Could you check a few things on this model? Use its own coordinates, in mm. A direction names the side the tool comes from. Coordinates: 2 decimals unless noted, no trailing zeros. Order: outer loops, then holes, each group sorted by start corner. A loop starts at its lowest first (then second) coordinate and runs counter-clockwise, first axis right, second up. Notation, with made-up numbers: (37.25, 1.25) -> (60.25, 1.25) arc R22 ccw to (60.25, 36.25) -> close; hole circle Ø4 at (23, -9). An arc over 180 degrees is marked (long way). Put each result on its own line as item: value. Start each with the question number.
Q1. Will these pins go through, and if not, where does the flat tip stop? pin 1 (6 mm diameter, centred on x = 15.5, y = -10.5, fed in from -Z); pin 2 (2 mm diameter, centred on y = -1, z = 1, fed in from -X); pin 3 (1.5 mm diameter, centred on x = 28, z = 0.5, fed in from -Y).
Q2. If we section it at A-A (y = 0): Please give me the cut outline in (x, z).
Q3. For faces 1 (the face through (-15, 7, 0)), 2 (the face through (0, 5, -5)), 3 (the face through (-15, -7, 0)), which set-ups out of +Z, -Z, +X, -X, +Y, -Y let a thin tool reach every point of the face, with its end or its side?
Q4. If we section it at B-B (x = -7.5): Please give me the cut outline in (y, z).
Q5. If we section it at D-D (x = 6.5): Please give me the cut outline in (y, z).
Q6. We'd pull the mould along X, two halves only. Please class faces 4 (the face through (-18, 7, 0)), 5 (the face through (39, 0, 0)), 6 (the face through (-7.605, -6.244, -0.275)): +X half, -X half, draft (parallel to the pull), parting line (faces both ways), or undercut.
Q7. If we section it at C-C (z = 0): Please give me the cut outline in (x, y).
Q8. Please list where these lines run through material, in increasing order: line 1 along X through (y, z) = (5, 5); line 2 along Y through (x, z) = (1.5, 1.5); line 3 along Y through (x, z) = (-16.5, 1.5).
from build123d import *

# Parameters (mm, degrees)
F8_DEPTH = 25


with BuildPart() as f2:
    # F1 (on Top) → F2 (revolve)
    with BuildSketch(Plane.XY):
        Polygon((0, 11), (0, 0), (39, 0), (39, 14), align=None)
    revolve(axis=Axis((3.167361, 0, 0), (1, 0, 0)))

    # F3 (on Top) → F4 (revolve)
    with BuildSketch(Plane.XY):
        Polygon((-15, 0), (0, 0), (0, 1.084316), (0, 6.25), (-15, 6.25), align=None)
    revolve(axis=Axis((-7.5, 0, 0), (-1, 0, 0)))

    # F5 (on Top) → F6 (revolve)
    with BuildSketch(Plane.XY):
        Polygon((-21, 0), (-15, 0), (-15, 8), (-21, 6), align=None)
    revolve(axis=Axis((-18, 0, 0), (-1, 0, 0)))

    # F7 (on Top) → F8 (cut, symmetric)
    with BuildSketch(Plane.XY):
        Polygon((-4.999509, 4.5511), (-23.682378, 4.5511), (-23.776263, 0), (-13.824584, 0), (-13.824584, 3.518378), align=None)
        Polygon((-13.824584, 0), (-23.776263, 0), (-23.682378, -4.5511), (-4.999509, -4.5511), (-13.824584, -3.518378), align=None)
    extrude(amount=F8_DEPTH, both=True, mode=Mode.SUBTRACT)


solid = f2.part
The answers:
1. pin 1: z = -9.63
1. pin 2: x = -13.82
1. pin 3: y = -13.21
2. outline: (-13.82, -6.25) -> (0, -6.25) -> (0, -11) -> (39, -14) -> (39, 14) -> (0, 11) -> (0, 6.25) -> (-13.82, 6.25) -> close
3. face 1: +Y
3. face 2: none
3. face 3: -Y
4. outline: (-4.55, -4.28) -> (-4.55, 4.28) arc R6.25 ccw to start; (-4.26, -4.57) arc R6.25 ccw to (4.26, -4.57) -> (4.26, 4.57) arc R6.25 ccw to (-4.26, 4.57) -> close; (4.55, -4.28) arc R6.25 ccw to (4.55, 4.28) -> close
5. outline: circle Ø23 at (0, 0)
6. face 4: -X half
6. face 5: +X half
6. face 6: undercut
7. outline: (-21, -6) -> (-15, -8) -> (-15, -6.25) -> (0, -6.25) -> (0, -11) -> (39, -14) -> (39, 14) -> (0, 11) -> (0, 6.25) -> (-15, 6.25) -> (-15, 8) -> (-21, 6) -> (-21, 4.55) -> (-5, 4.55) -> (-13.82, 3.52) -> (-13.82, -3.52) -> (-5, -4.55) -> (-21, -4.55) -> close
8. line 1: -17.79 to -15, 0 to 39
8. line 2: -11.01 to 11.01
8. line 3: -7.35 to -4.55, 4.55 to 7.35
